Drawing for the job (mm, zero at the part's lowest x, y, z). A direction names the side the tool comes from. Round coordinates to 2 decimals unless told otherwise and drop trailing zeros. Write each loop counter-clockwise with the first axis right and the second up, starting at its lowest first coordinate (ties: lowest second). Pieces come first, ordered by that corner, then holes. Notation, with made-up numbers: (72.25, 14) -> (89.25, 14) arc R32 ccw to (89.25, 40) -> close; hole circle Ø5 at (60, 7). An arc over 180 degrees is marked (long way). Answer in a Markdown table with one row per item. Add a question column.
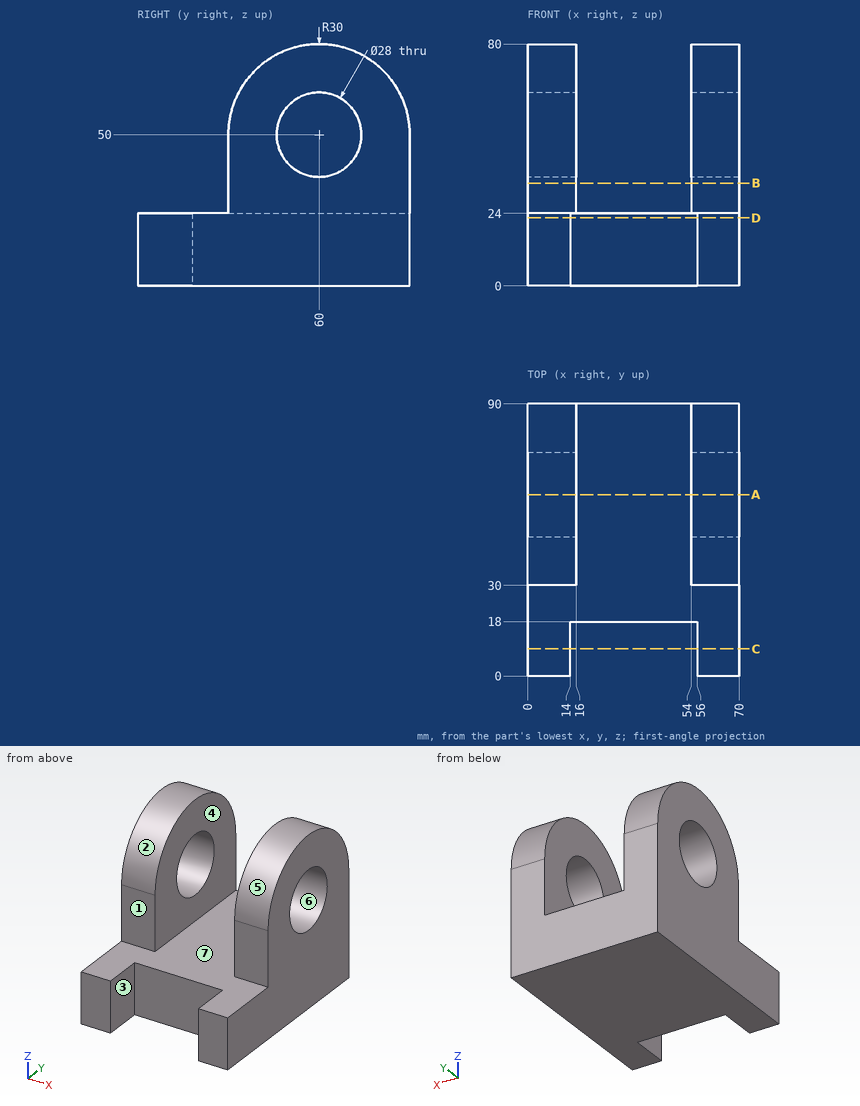
(1) Drop flat-ended pins along their axis: P1, Ø17, axis at y = 59, z = 42.5, coming from the -X side; P2, Ø7, axis at x = 43.5, z = 12.5, coming from the -Y side; P3, Ø21, axis at x = 34, y = 56.5, coming from the +Z side. Give the stop position or say it passes through.
(2) Saw through at A-A (y = 60). List the corners of the cut face in (x, z), plus the area to 3 significant figures.
(3) Saw through at C-C (y = 9). List the corners of the cut face in (x, z), plus the area to 3 significant figures.
(4) Probe line 1 along Z through (x, y) = (62.5, 60); line 2 along Y through (x, z) = (9, 50); line 3 along X through (y, z) = (75.5, 63). List the from-to ranges inside material, lowest first.
(5) Which spindle directions (+Z, -Z, +X, -X, +Y, -Y) get a long thin tool onto all of the face, cutting with end or side? Do the marked faces 1, 2, 3 and 4. Say none if no direction does.
(6) Mould opens along Y. For the marked faces 5, 6 and 7 say: pulls with the +Y half, pulls with the -Y half, needs draft (parallel to the pull), parting line crosses it, or undercut.
(7) Saw through at D-D (z = 22.5). List the corners of the cut face in (x, y), plus the area to 3 significant figures.
(8) Saw through at B-B (z = 34). List the corners of the cut face in (x, y).
Answer sheet:
| question | item | result |
|---|---|---|
| 1 | P1 | stops at x = 0 |
| 1 | P2 | stops at y = 18 |
| 1 | P3 | stops at z = 24 |
| 2 | outline | (0, 0) -> (70, 0) -> (70, 36) -> (54, 36) -> (54, 24) -> (16, 24) -> (16, 36) -> (0, 36) -> close; (0, 64) -> (16, 64) -> (16, 80) -> (0, 80) -> close; (54, 64) -> (70, 64) -> (70, 80) -> (54, 80) -> close |
| 2 | area | 2,580 mm² |
| 3 | outline | (0, 0) -> (14, 0) -> (14, 24) -> (0, 24) -> close; (56, 0) -> (70, 0) -> (70, 24) -> (56, 24) -> close |
| 3 | area | 672 mm² |
| 4 | line 1 | z = 0 to 36, 64 to 80 |
| 4 | line 2 | y = 30 to 46, 74 to 90 |
| 4 | line 3 | x = 0 to 16, 54 to 70 |
| 5 | face 1 | +Z, +X, -X, -Y |
| 5 | face 2 | +Z, +X, -X |
| 5 | face 3 | +Z, -Z, -Y |
| 5 | face 4 | +Z, +Y, -Y |
| 6 | face 5 | parting line crosses it |
| 6 | face 6 | undercut |
| 6 | face 7 | needs draft |
| 7 | outline | (0, 0) -> (14, 0) -> (14, 18) -> (56, 18) -> (56, 0) -> (70, 0) -> (70, 90) -> (0, 90) -> close |
| 7 | area | 5,540 mm² |
| 8 | outline | (0, 30) -> (16, 30) -> (16, 90) -> (0, 90) -> close; (54, 30) -> (70, 30) -> (70, 90) -> (54, 90) -> close |
